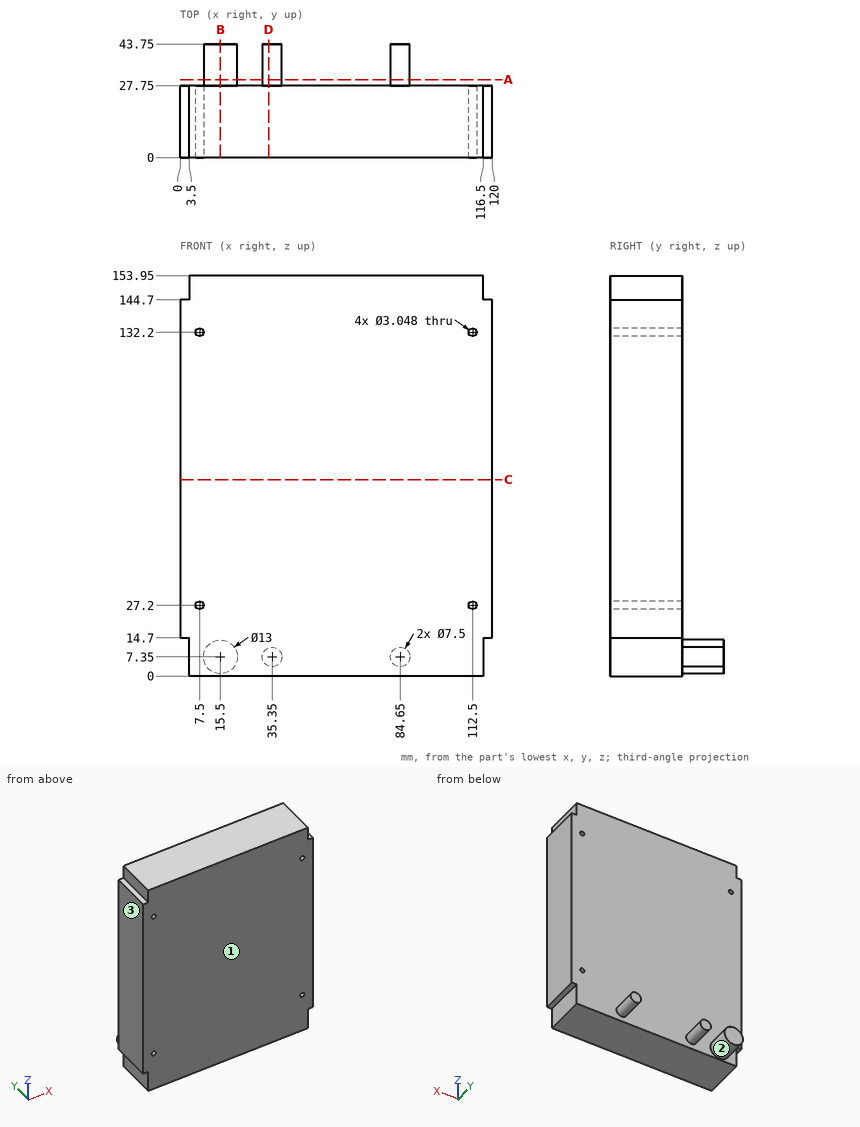
Drawing for the job (mm, zero at the part's lowest x, y, z). Give positions to 0.01 mm unless a question says otherwise; leave off trailing zeros. Order: outer loops, then holes, each group sorted by start corner. A loop starts at its lowest first (then second) coordinate and runs counter-clockwise, first axis right, second up. Notation, with made-up numbers: (80.25, 20.25) - (115.25, 20.25) arc R21 ccw to (115.25, 39.25) - close; hole circle Ø1 at (49.5, 73). An arc over 180 degrees is marked (long way). Write item = value, one per line. Start each with the question number.
1. Two-plate mould, pull along X, no slides. Class the marked faces 1, 2 and 3: pulls with the +X half, pulls with the -X half, needs draft (parallel to the pull), parting line crosses it, or undercut.
2. Probe line 1 along Z through (x, y) = (7.5, 9.25); line 2 along X through (y, z) = (14, 27); line 3 along Z through (x, y) = (7, 19). List the from-to ranges inside material, lowest first.
3. Cut at A-A, the plane y = 30. List the corners of the cut face in (x, z), and give its area (3 significant figures).
4. Drop flat-ended pins along their axis: P1, Ø1.8, axis at x = 1.5, y = 11.5, coming from the -Z side; P2, Ø1.8, axis at x = 118.5, y = 19.5, coming from the +Z side; P3, Ø10, axis at y = 19.5, z = 150, coming from the +X side. Give the stop position or say it passes through.
5. Cut at B-B, the plane x = 15.5. List the corners of the cut face in (y, z).
6. Cut at D-D, the plane x = 34. List the corners of the cut face in (y, z).
7. Cut at C-C, the plane z = 75.5. List the corners of the cut face in (x, y), and give its area (3 significant figures).
Taken from the geometry:
q1.face_1 = needs draft
q1.face_2 = undercut
q1.face_3 = pulls with the -X half
q2.line_1 = 0 to 25.68, 28.72 to 130.68, 133.72 to 153.95
q2.line_2 = 0 to 5.99, 9.01 to 110.99, 114.01 to 120
q2.line_3 = 0 to 25.76, 28.64 to 130.76, 133.64 to 153.95
q3.outline = circle Ø13 at (15.5, 7.35); circle Ø7.5 at (35.35, 7.35); circle Ø7.5 at (84.65, 7.35)
q3.area = 221 mm²
q4.P1 = 14.7
q4.P2 = 144.7
q4.P3 = 116.5
q5.outline = (0, 0) - (27.75, 0) - (27.75, 0.85) - (43.75, 0.85) - (43.75, 13.85) - (27.75, 13.85) - (27.75, 153.95) - (0, 153.95) - close
q6.outline = (0, 0) - (27.75, 0) - (27.75, 3.85) - (43.75, 3.85) - (43.75, 10.85) - (27.75, 10.85) - (27.75, 153.95) - (0, 153.95) - close
q7.outline = (0, 0) - (120, 0) - (120, 27.75) - (0, 27.75) - close
q7.area = 3,330 mm²
